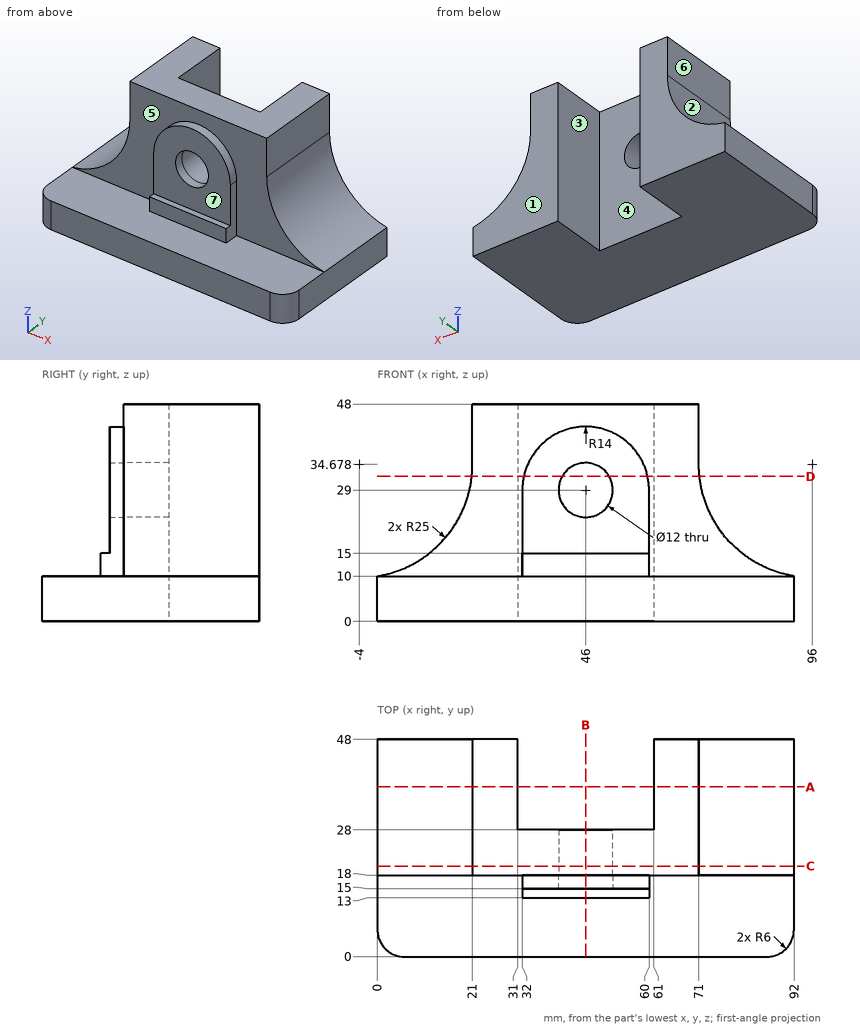
Check sheet for the drawn part. Datum: minimum x, y, z corner. Units: mm. A direction names the side the tool comes from. Give positions to 0.01 mm unless a question says otherwise; leave off trailing zeros. Loops run counter-clockwise (first coordinate to the right, second up) from the corner with the lowest first, then second, coordinate; pieces in that order, holes last. Notation, with made-up numbers: M -14.75,20.25 L 37.25,20.25 A27 cw 37.25,47.25 Z; hole C 55,4 d2. An arc over 180 degrees is marked long. Answer as CSV lines item,"result".
Item 1: Draft check along X on the marked faces 1, 2 and 3. Enter one of: pulls with the +X half, pulls with the -X half, needs draft (parallel to the pull), parting line crosses it, or undercut.
Reply:
face 1,"needs draft"
face 2,"pulls with the -X half"
face 3,"undercut"
Item 2: Sectioned sample at C-C, the plane y = 20. Enter the section's corners in (x, z).
Reply:
outline,"M 0,0 L 92,0 L 92,10 A25 cw 71,34.68 L 71,48 L 21,48 L 21,34.68 A25 cw 0,10 Z; hole C 46,29 d12"
Item 3: Scan lines: L1, parallel to Z at x = 46, y = 16.3; L2, parallel to Z at x = 46, y = 20; L3, parallel to Y at x = 8, z = 11. Record each from-to range of solid material in increasing order.
Reply:
L1,"0 to 23, 35 to 43"
L2,"0 to 23, 35 to 48"
L3,"18 to 48"
Item 4: Sectioned sample at D-D, the plane z = 32. Enter the section's corners in (x, y), then the cut area to 3 significant figures.
Reply:
outline,"M 20.86,18 L 32.33,18 L 32.33,15 L 40.8,15 L 40.8,28 L 31,28 L 31,48 L 20.86,48 Z; M 51.2,15 L 59.67,15 L 59.67,18 L 71.14,18 L 71.14,48 L 61,48 L 61,28 L 51.2,28 Z"
area,"856 mm^2"
Item 5: Depth check by flat-ended pin: pin 1 Ø1 at (y, z) = (39.5, 34) entering from -X; pin 2 Ø14.5 at (y, z) = (35.5, 42) entering from +X; pin 3 Ø9 at (x, z) = (48.5, 21.5) entering from +Y. Enter the tip coordinate at first touch or a pass-through.
Reply:
pin 1,"x = 20.97"
pin 2,"x = 71"
pin 3,"y = 28"
Item 6: Set-up check for the marked faces 4, 5, 6 and 7: record each of +Z, -Z, +X, -X, +Y, -Y from which the full face is reachable in a straight line by a thin tool's end or side.
Reply:
face 4,"+Z, -Z, +Y"
face 5,"+Z, -Y"
face 6,"+Z, -X, +Y, -Y"
face 7,"+Z, +X, -X, -Y"
Item 7: Sectioned sample at B-B, the plane x = 46. Enter the section's corners in (y, z), then the cut area to 3 significant figures.
Reply:
outline,"M 0,0 L 28,0 L 28,23 L 15,23 L 15,15 L 13,15 L 13,10 L 0,10 Z; M 15,35 L 28,35 L 28,48 L 18,48 L 18,43 L 15,43 Z"
area,"613 mm^2"
Item 8: Sectioned sample at A-A, the plane y = 37.5. Enter the section's corners in (x, z).
Reply:
outline,"M 0,0 L 31,0 L 31,48 L 21,48 L 21,34.68 A25 cw 0,10 Z; M 61,0 L 92,0 L 92,10 A25 cw 71,34.68 L 71,48 L 61,48 Z"
